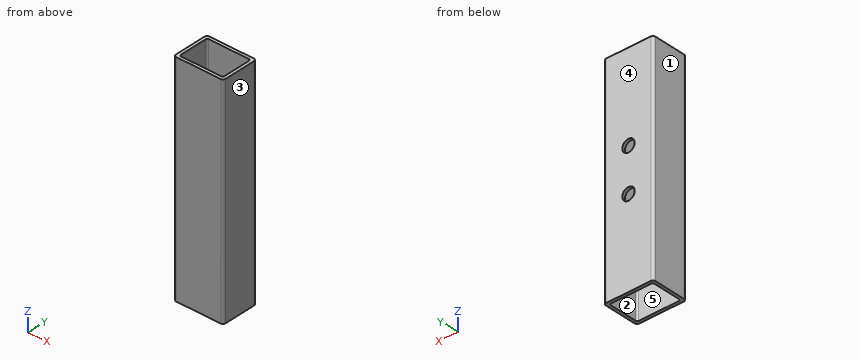
from build123d import *

# Parameters (mm, degrees)
BOSS_EXTRUDE1_DEPTH = 225.425
SKETCH9_R           = 6.35
CUT_EXTRUDE2_DEPTH  = 3.048


with BuildPart() as part:
    # Sketch4 → Boss-Extrude1 (new body)
    with BuildSketch(Plane.XY):
        with BuildLine():
            Line((25.4, -16.51), (25.4, 16.51))
            ThreePointArc((25.4, 16.51), (24.656051224, 18.306051224), (22.86, 19.05))
            Line((22.86, 19.05), (-22.86, 19.05))
            ThreePointArc((-22.86, 19.05), (-24.656051224, 18.306051224), (-25.4, 16.51))
            Line((-25.4, 16.51), (-25.4, -16.51))
            ThreePointArc((-25.4, -16.51), (-24.656051224, -18.306051224), (-22.86, -19.05))
            Line((-22.86, -19.05), (22.86, -19.05))
            ThreePointArc((22.86, -19.05), (24.656051224, -18.306051224), (25.4, -16.51))
        make_face()
        with BuildLine():
            Line((22.352, 14.4018), (22.352, -14.4018))
            ThreePointArc((22.352, -14.4018), (21.883312271, -15.533312271), (20.7518, -16.002))
            Line((20.7518, -16.002), (-20.7518, -16.002))
            ThreePointArc((-20.7518, -16.002), (-21.883312271, -15.533312271), (-22.352, -14.4018))
            Line((-22.352, -14.4018), (-22.352, 14.4018))
            ThreePointArc((-22.352, 14.4018), (-21.883312271, 15.533312271), (-20.7518, 16.002))
            Line((-20.7518, 16.002), (20.7518, 16.002))
            ThreePointArc((20.7518, 16.002), (21.883312271, 15.533312271), (22.352, 14.4018))
        make_face(mode=Mode.SUBTRACT)
    extrude(amount=BOSS_EXTRUDE1_DEPTH)

    # Sketch9 → Cut-Extrude2 (cut)
    with BuildSketch(Plane(origin=(0, 19.05, 0), x_dir=(1, 0, 0), z_dir=(0, 1, 0))):
        with Locations(Location((0, -134.9375, 0), (0, 0, 270))):
            Circle(SKETCH9_R)
        with Locations(Location((0, -90.4875, 0), (0, 0, 270))):
            Circle(SKETCH9_R)
    extrude(amount=-CUT_EXTRUDE2_DEPTH, mode=Mode.SUBTRACT)


solid = part.part
Verification items for the finished model (mm, model axes). Face numbers are marked on the shaded views. A direction names the side the tool comes from. Coordinates: 2 decimals unless noted, no trailing zeros. Order: outer loops, then holes, each group sorted by start corner. A loop starts at its lowest first (then second) coordinate and runs counter-clockwise, first axis right, second up. Notation, with made-up numbers: M 37,38.25 L 61,38.25 A19 ccw 61,62.25 Z; hole C 60.5,57 d7. An arc over 180 degrees is marked long. Return JSON: item names as keys, results as strings.
1) Cross-section at B-B, the plane y = -1. Record the boundary of the cut face in (x, z) (3 decimals), and give its area (3 significant figures).
Answer list:
{"outline": "M -25.4,0 L -22.352,0 L -22.352,225.425 L -25.4,225.425 Z; M 22.352,0 L 25.4,0 L 25.4,225.425 L 22.352,225.425 Z", "area": "1,370 mm2"}
2) Access from +Z, -Z, +X, -X, +Y, -Y to the whole of each face (thin tool, end or side, straight path). Record for the marked faces 1 and 2.
Answer list:
{"face 1": "+Z, -Z, -X, +Y, -Y", "face 2": "+Z, -Z"}
3) Thickness scan on L1, parallel to Y at x = 17, z = 33; L2, parallel to X at y = 1, z = 123; L3, parallel to X at y = -15.5, z = 68. Record the ranges inside material, lowest first. Write a range as [from, to].
Answer list:
{"L1": "[-19.05, -16], [16, 19.05]", "L2": "[-25.4, -22.35], [22.35, 25.4]", "L3": "[-25.4, -21.92], [21.92, 25.4]"}
4) Cross-section at C-C, the plane x = 17.5. Record the boundary of the cut face in (y, z) (3 decimals).
Answer list:
{"outline": "M -19.05,0 L -16.002,0 L -16.002,225.425 L -19.05,225.425 Z; M 16.002,0 L 19.05,0 L 19.05,225.425 L 16.002,225.425 Z"}
5) Cross-section at A-A, the plane x = 0. Count the separate pieces of the cut face and the enclosed holes in it, and give its area (3 significant figures).
Answer list:
{"separate pieces": "4", "enclosed holes": "0", "area": "1,300 mm2"}
6) Release check for a two-part mould opening along X. For the marked faces 3, 4 and 5 record: +X half, -X half, draft (parallel to the pull), parting line (faces both ways), or undercut.
Answer list:
{"face 3": "+X half", "face 4": "draft", "face 5": "undercut"}
7) Cross-section at D-D, the plane z = 125. Record the boundary of the cut face in (x, y), and give its area (3 significant figures).
Answer list:
{"outline": "M -25.4,-16.51 A2.54 ccw -22.86,-19.05 L 22.86,-19.05 A2.54 ccw 25.4,-16.51 L 25.4,16.51 A2.54 ccw 22.86,19.05 L -22.86,19.05 A2.54 ccw -25.4,16.51 Z; hole M -22.35,-14.4 A1.6 ccw -20.75,-16 L 20.75,-16 A1.6 ccw 22.35,-14.4 L 22.35,14.4 A1.6 ccw 20.75,16 L -20.75,16 A1.6 ccw -22.35,14.4 Z", "area": "501 mm2"}
8) Gauge pin test, flat ends, axial feed: pin 1 (11.5 mm diameter, centred on x = 0, z = 134.94, fed in from +Y); pin 2 (3 mm diameter, centred on x = -19.5, y = -11, fed in from +Z). Record the tip position at first contact, or that the pin passes through.
Answer list:
{"pin 1": "y = -16", "pin 2": "through"}
